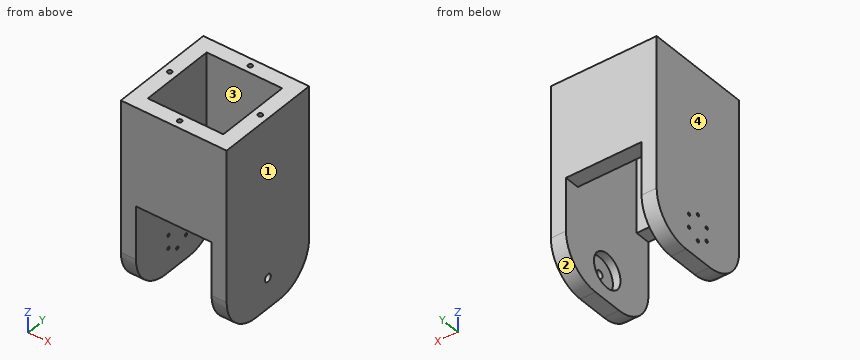
from build123d import *

# Parameters (mm, degrees)
SKETCH_1_W           = 140
SKETCH_1_H           = 140
SKETCH_1_W_2         = 100
SKETCH_1_H_2         = 100
EXTRUDE_3_DEPTH      = 250
SKETCH_2_W           = 100
SKETCH_2_H           = 140
CUT_EXTRUDE_1_DEPTH  = 120
SKETCH_4_R           = 15.704370783
SKETCH_4_R_2         = 3
CUT_EXTRUDE_2_DEPTH  = 10
SKETCH_8_R           = 2
CUT_EXTRUDE_3_DEPTH  = 20
FILLET_1_R           = 50
SKETCH_10_R          = 22.5
CUT_EXTRUDE_4_DEPTH  = 10
SKETCH_11_R          = 5
CUT_EXTRUDE_10_DEPTH = 12


with BuildPart() as part:
    # 草图1 → 凸台-拉伸3 (new body)
    with BuildSketch(Plane.XY):
        with Locations((-127.289473684, 36.657894737)):
            Rectangle(SKETCH_1_W, SKETCH_1_H)
        with Locations((-127.289473684, 36.657894737)):
            Rectangle(SKETCH_1_W_2, SKETCH_1_H_2, mode=Mode.SUBTRACT)
    extrude(amount=EXTRUDE_3_DEPTH)

    # 草图2 → 切除-拉伸1 (cut)
    with BuildSketch(Plane(origin=(0, 0, 0), x_dir=(-1, 0, 0), z_dir=(0, 0, -1))):
        with Locations((127.289473684, 36.657894737)):
            Rectangle(SKETCH_2_W, SKETCH_2_H)
    extrude(amount=-CUT_EXTRUDE_1_DEPTH, mode=Mode.SUBTRACT)

    # 草图4 → 切除-拉伸2 (cut)
    with BuildSketch(Plane.XY.offset(250)):
        with Locations((-127.289473684, 36.657894737)):
            Circle(SKETCH_4_R)
        with Locations((-187.289473684, 36.657894737)):
            Circle(SKETCH_4_R_2)
        with Locations((-127.289473684, 96.657894737)):
            Circle(SKETCH_4_R_2)
        with Locations((-67.289473684, 36.657894737)):
            Circle(SKETCH_4_R_2)
        with Locations((-127.289473684, -23.342105263)):
            Circle(SKETCH_4_R_2)
    extrude(amount=-CUT_EXTRUDE_2_DEPTH, mode=Mode.SUBTRACT)

    # 草图8 → 切除-拉伸3 (cut)
    with BuildSketch(Plane.ZY.offset(197.289473684)):
        with Locations((22.75, 36.657894737)):
            Circle(SKETCH_8_R)
        with Locations((31.375, 51.596832952)):
            Circle(SKETCH_8_R)
        with Locations((48.625, 51.596832952)):
            Circle(SKETCH_8_R)
        with Locations((57.25, 36.657894737)):
            Circle(SKETCH_8_R)
        with Locations((48.625, 21.718956522)):
            Circle(SKETCH_8_R)
        with Locations((31.375, 21.718956522)):
            Circle(SKETCH_8_R)
    extrude(amount=-CUT_EXTRUDE_3_DEPTH, mode=Mode.SUBTRACT)

    # 圆角1
    fillet_1_edges = [part.edges().sort_by_distance(p)[0] for p in [
        (-67.289473684, -33.342105263, 0),
        (-187.289473684, 106.657894737, 0),
        (-187.289473684, -33.342105263, 0),
        (-67.289473684, 106.657894737, 0),
    ]]
    fillet(fillet_1_edges, radius=FILLET_1_R)

    # 草图10 → 切除-拉伸4 (cut)
    with BuildSketch(Plane.ZY.offset(77.289473684)):
        with Locations((40, 36.657894737)):
            Circle(SKETCH_10_R)
    extrude(amount=-CUT_EXTRUDE_4_DEPTH, mode=Mode.SUBTRACT)

    # 草图11 → 切除-拉伸10 (cut)
    with BuildSketch(Plane.ZY.offset(67.289473684)):
        with Locations((40, 36.657894737)):
            Circle(SKETCH_11_R)
    extrude(amount=-CUT_EXTRUDE_10_DEPTH, mode=Mode.SUBTRACT)


solid = part.part
Design review of the part built by this model. Coordinates are the model's own, in mm. Face numbers are marked on the shaded views. Round coordinates to 2 decimals unless told otherwise and drop trailing zeros. Write each loop counter-clockwise with the first axis right and the second up, starting at its lowest first coordinate (ties: lowest second). Pieces come first, ordered by that corner, then holes. Notation, with made-up numbers: (-3, 24) - (51, 24) arc R11 ccw to (51, 44) - close; hole circle Ø1 at (33.25, 21.5). An arc over 180 degrees is marked (long way). Use a Markdown table: item, result. Add a question column.
1. We need section B-B (z = 91). State the section outline as (x, y) points, then the cut area to 3 significant figures.
2. We need section A-A (x = -138). State the section outline as (y, z) points, then the cut area to 3 significant figures.
3. Wall thickness on probe 1 along X at (y, z) = (28.5, 231); probe 2 along Y at (x, z) = (-170.5, 147.5); probe 3 along Z at (x, y) = (-162, 97): over which ranges is each line inside the solid? List them lowest first.
4. We need section C-C (z = 168). State the section outline as (x, y) points.
5. Clearance check with flat-ended pins moving along their axes: pin 1 (2.5 mm diameter, centred on y = 51.6, z = 48.62, fed in from -X); pin 2 (8 mm diameter, centred on x = -127.29, y = 96.66, fed in from -Z); pin 3 (3.5 mm diameter, centred on x = -67.29, y = 36.66, fed in from +Z). State where each tip first meets the part, or that it passes through.
6. Mouldability with a two-part tool opening along X and no side actions: class the marked faces 1, 2, 3 and 4 as +X half, -X half, draft (parallel to the pull), parting line (faces both ways), or undercut.
7. We need section D-D (z = 40). State the section outline as (x, y) points.
Output:
| question | item | result |
|---|---|---|
| 1 | outline | (-197.29, -33.34) - (-177.29, -33.34) - (-177.29, 106.66) - (-197.29, 106.66) - close; (-77.29, -33.34) - (-57.29, -33.34) - (-57.29, 106.66) - (-77.29, 106.66) - close |
| 1 | area | 5,600 mm2 |
| 2 | outline | (-33.34, 120) - (-13.34, 120) - (-13.34, 250) - (-33.34, 250) - close; (86.66, 120) - (106.66, 120) - (106.66, 250) - (86.66, 250) - close |
| 2 | area | 5,200 mm2 |
| 3 | probe 1 | x = -197.29 to -177.29, -77.29 to -57.29 |
| 3 | probe 2 | y = -33.34 to -13.34, 86.66 to 106.66 |
| 3 | probe 3 | z = 120 to 250 |
| 4 | outline | (-197.29, -33.34) - (-57.29, -33.34) - (-57.29, 106.66) - (-197.29, 106.66) - close; hole (-177.29, -13.34) - (-77.29, -13.34) - (-77.29, 86.66) - (-177.29, 86.66) - close |
| 5 | pin 1 | stops at x = -67.29 |
| 5 | pin 2 | stops at z = 120 |
| 5 | pin 3 | stops at z = 240 |
| 6 | face 1 | +X half |
| 6 | face 2 | draft |
| 6 | face 3 | undercut |
| 6 | face 4 | -X half |
| 7 | outline | (-197.29, -32.33) - (-177.29, -32.33) - (-177.29, 105.65) - (-197.29, 105.65) - close; (-77.29, -32.33) - (-57.29, -32.33) - (-57.29, 31.66) - (-67.29, 31.66) - (-67.29, 14.16) - (-77.29, 14.16) - close; (-77.29, 59.16) - (-67.29, 59.16) - (-67.29, 41.66) - (-57.29, 41.66) - (-57.29, 105.65) - (-77.29, 105.65) - close |
